Read the model definition and answer for the solid it produces. Units are mm, in the model's axes. Face numbers are marked on the shaded views. A direction names the side the tool comes from. Coordinates: 2 decimals unless noted, no trailing zeros. Order: outer loops, then holes, each group sorted by start corner. A loop starts at its lowest first (then second) coordinate and runs counter-clockwise, first axis right, second up. Notation, with made-up numbers: (-2.75, 3) - (9.25, 3) arc R15 ccw to (9.25, 19) - close; hole circle Ø9 at (64, 39.5). An arc over 180 degrees is marked (long way). Use one line per item in the form item = value.
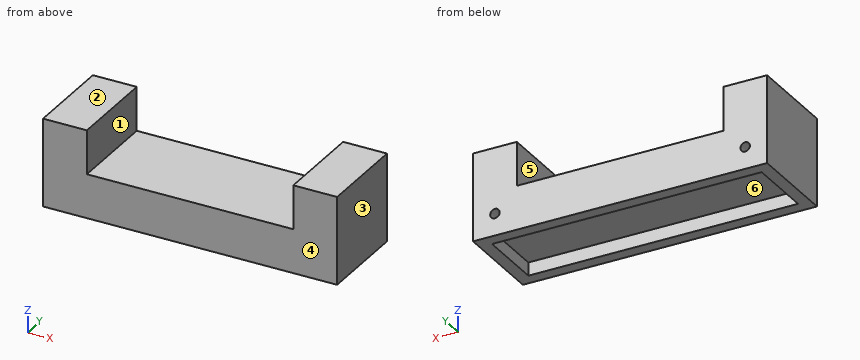
```python
from build123d import *

# Parameters (mm, degrees)
SKETCH_W        = 134.142136
SKETCH_H        = 41.142136
PAD_DEPTH       = 20
SKETCH001_W     = 20
SKETCH001_H     = 41.142136
PAD001_DEPTH    = 20
SKETCH002_W     = 123
SKETCH002_H     = 30
POCKET_DEPTH    = 6
SKETCH003_R     = 2.1463
POCKET001_DEPTH = 10


with BuildPart() as part:
    # Sketch → Pad (new body)
    with BuildSketch(Plane.XY):
        Rectangle(SKETCH_W, SKETCH_H)
    extrude(amount=PAD_DEPTH)

    # Sketch001 (on Face6 of Pad) → Pad001 (join)
    with BuildSketch(Plane.XY.offset(20)):
        with Locations((-57.071068, 0)):
            Rectangle(SKETCH001_W, SKETCH001_H)
        with Locations((57.071068, 0)):
            Rectangle(SKETCH001_W, SKETCH001_H)
    extrude(amount=PAD001_DEPTH)

    # Sketch002 (on Face4 of Pad001) → Pocket (cut)
    with BuildSketch(Plane(origin=(0, 0, 0), x_dir=(1, 0, 0), z_dir=(0, 0, -1))):
        Rectangle(SKETCH002_W, SKETCH002_H)
    extrude(amount=-POCKET_DEPTH, mode=Mode.SUBTRACT)

    # Sketch003 (on Face1 of Pocket) → Pocket001 (cut)
    with BuildSketch(Plane(origin=(0, 20.571068, 0), x_dir=(-1, 0, 0), z_dir=(0, 1, 0))):
        with Locations((-57.071068, 10)):
            Circle(SKETCH003_R)
        with Locations((57.071068, 10)):
            Circle(SKETCH003_R)
    extrude(amount=-POCKET001_DEPTH, mode=Mode.SUBTRACT)


solid = part.part
```
(1) Straight lines are drawn through the part: L1, parallel to X at y = 18.5, z = 35; L2, parallel to Y at x = 2.5, z = 2; L3, parallel to Z at x = -23.5, y = 12.5. For each, find the intervals that lie inside material, in ascending order.
Answer list:
L1 = -67.07 to -47.07, 47.07 to 67.07
L2 = -20.57 to -15, 15 to 20.57
L3 = 6 to 20
(2) Section D-D, the plane x = -20.5 is taken. Write down the section's boundary in (y, z), then the cut area to 3 significant figures.
Answer list:
outline = (-20.57, 0) - (-15, 0) - (-15, 6) - (15, 6) - (15, 0) - (20.57, 0) - (20.57, 20) - (-20.57, 20) - close
area = 643 mm2
(3) Which of the six approach directions +Z, -Z, +X, -X, +Y, -Y give full straight-line access (tool end or side, diameter ignored) to the marked faces 4, 5 and 6?
Answer list:
face_4 = +Z, -Z, +X, -X, -Y
face_5 = +Z, +Y, -Y
face_6 = -Z
(4) Section A-A, the plane y = 18 is taken. Write down the section's boundary in (x, z), then the cut area to 3 significant figures.
Answer list:
outline = (-67.07, 0) - (67.07, 0) - (67.07, 40) - (47.07, 40) - (47.07, 20) - (-47.07, 20) - (-47.07, 40) - (-67.07, 40) - close; hole circle Ø4.29 at (-57.07, 10); hole circle Ø4.29 at (57.07, 10)
area = 3,450 mm2
(5) Given pin 1 Ø2 at (x, z) = (57.5, 9.5) entering from +Y; pin 2 Ø9 at (x, y) = (-27, 0.5) entering from -Z; pin 3 Ø5 at (x, y) = (-34, 11) entering from +Z, each flat-ended and moving along its own axis, determine where each tip first touches the part or whether it passes through.
Answer list:
pin_1 = 10.57
pin_2 = 6
pin_3 = 20
(6) Section C-C, the plane y = 4 is taken. Write down the section's boundary in (x, z).
Answer list:
outline = (-67.07, 0) - (-61.5, 0) - (-61.5, 6) - (61.5, 6) - (61.5, 0) - (67.07, 0) - (67.07, 40) - (47.07, 40) - (47.07, 20) - (-47.07, 20) - (-47.07, 40) - (-67.07, 40) - close
(7) The mould has two halves that part along X. Classify the marked faces 1, 2 and 3: +X half, -X half, draft (parallel to the pull), parting line (faces both ways), or undercut.
Answer list:
face_1 = undercut
face_2 = draft
face_3 = +X half
(8) Section B-B, the plane z = 37 is taken. Write down the section's boundary in (x, y).
Answer list:
outline = (-67.07, -20.57) - (-47.07, -20.57) - (-47.07, 20.57) - (-67.07, 20.57) - close; (47.07, -20.57) - (67.07, -20.57) - (67.07, 20.57) - (47.07, 20.57) - close
